```python
from build123d import *

# Parameters (mm, degrees)
SKETCH1_R           = 6
BOSS_EXTRUDE1_DEPTH = 10
SKETCH2_R           = 11.75
BOSS_EXTRUDE2_DEPTH = 3
FILLET1_R           = 0.5


with BuildPart() as part:
    # Sketch1 → Boss-Extrude1 (new body)
    with BuildSketch(Plane(origin=(0, 0, 0), x_dir=(1, 0, 0), z_dir=(0, 1, 0))):
        Polygon((10.392304845, 0), (5.196152423, 9), (-5.196152423, 9), (-10.392304845, 0), (-5.196152423, -9), (5.196152423, -9), align=None)
        with Locations(Location((0, 0, 0), (0, 0, 270))):
            Circle(SKETCH1_R, mode=Mode.SUBTRACT)
    extrude(amount=BOSS_EXTRUDE1_DEPTH)

    # Sketch2 → Boss-Extrude2 (add)
    with BuildSketch(Plane.XZ):
        with Locations(Location((0, 0, 0), (0, 0, 270))):
            Circle(SKETCH2_R)
        Polygon((10.392304845, 0), (5.196152423, 9), (-5.196152423, 9), (-10.392304845, 0), (-5.196152423, -9), (5.196152423, -9), align=None, mode=Mode.SUBTRACT)
    extrude(amount=-BOSS_EXTRUDE2_DEPTH)

    # Sketch3 → Cut-Revolve1 (revolve, cut)
    with BuildSketch(Plane.XY, mode=Mode.PRIVATE) as cut_revolve1_sk:
        Polygon((-10.392304845, 9), (-9.392304845, 10), (-10.392304845, 10), align=None)
        Polygon((-10.392304845, 3), (-11.75, 2.5), (-11.75, 3), align=None)
    revolve(cut_revolve1_sk.sketch.rotate(Axis((0, 0, 0), (0, 1, 0)), 270), axis=Axis((0, 0, 0), (0, 1, 0)), mode=Mode.SUBTRACT)

    # Fillet1
    fillet1_edges = [part.edges().sort_by_distance(p)[0] for p in [
        (0, 0, 11.75),
        (0, 2.5, 11.75),
    ]]
    fillet(fillet1_edges, radius=FILLET1_R)


solid = part.part
```
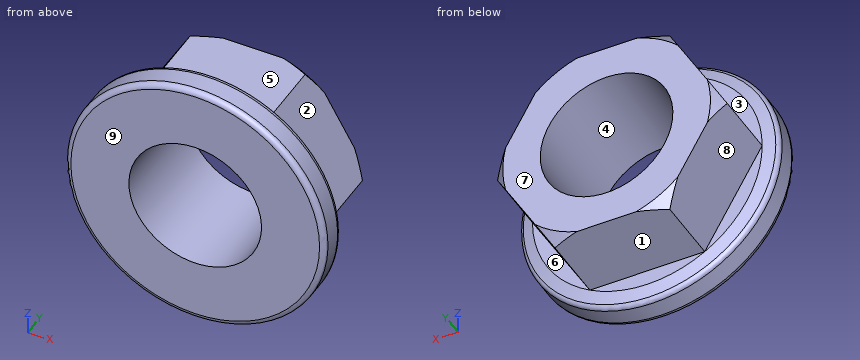
Could you check a few things on this model? Use its own coordinates, in mm. Face numbers are marked on the shaded views. A direction names the side the tool comes from. Coordinates: 2 decimals unless noted, no trailing zeros. Write each loop counter-clockwise with the first axis right and the second up, starting at its lowest first coordinate (ties: lowest second). Pieces come first, ordered by that corner, then holes. Notation, with made-up numbers: (79.25, 0.5) -> (133.25, 0.5) arc R20 ccw to (133.25, 7.5) -> close; hole circle Ø7 at (63, 47). An arc over 180 degrees is marked (long way). Return JSON: item names as keys, results as strings.
(1) Which directions (+Z, -Z, +X, -X, +Y, -Y) give clear straight access to the entire face, cutting with the end or side of a thin tool? Please do the marked faces 5, 6, 7, 8 and 9.
Numbers:
{"face 5": "+Z, +X, -X, +Y", "face 6": "-Z, +X, +Y", "face 7": "+Z, -Z, +X, -X, +Y", "face 8": "-Z, -X, +Y", "face 9": "+Z, -Z, +X, -X, -Y"}
(2) Imagine slicing it at A-A, the plane y = 5.75. Please give me the cut outline in (x, z), then the cut area to 3 significant figures.
Numbers:
{"outline": "(-10.39, 0) -> (-5.2, -9) -> (5.2, -9) -> (10.39, 0) -> (5.2, 9) -> (-5.2, 9) -> close; hole circle Ø12 at (0, 0)", "area": "167 mm2"}
(3) I need wall thicknesses on L1, parallel to Y at x = 0.5, z = 9.5; L2, parallel to X at y = 7.5, z = 4.75; L3, parallel to Z at x = 1.25, y = 9.75. Which ranges of each line are inside material? Lowest first, please.
Numbers:
{"L1": "y = 0 to 3", "L2": "x = -7.65 to -3.67, 3.67 to 7.65", "L3": "z = -9 to -5.87, 5.87 to 9"}
(4) We'd pull the mould along Z, two halves only. Please class the marked faces 1, 2, 3 and 4: +Z half, -Z half, draft (parallel to the pull), parting line (faces both ways), or undercut.
Numbers:
{"face 1": "-Z half", "face 2": "+Z half", "face 3": "draft", "face 4": "undercut"}
(5) I'm going to push flat-ended pins straight in: pin 1 (1 mm diameter, centred on x = -6, z = -6.5, fed in from -Y); pin 2 (3.5 mm diameter, centred on x = 0.5, y = 5, fed in from -Z); pin 3 (1.5 mm diameter, centred on y = 5.5, z = 9, fed in from +X); pin 4 (2 mm diameter, centred on x = -2.5, y = 7.5, fed in from +Z). Where does each tip first touch, or does it pass through?
Numbers:
{"pin 1": "stops at y = 0", "pin 2": "stops at z = -9", "pin 3": "stops at x = 5.63", "pin 4": "stops at z = 9"}
